Here's how the part is built. I have some questions about the finished solid (model axes, mm). Round coordinates to 2 decimals unless told otherwise and drop trailing zeros. Write each loop counter-clockwise with the first axis right and the second up, starting at its lowest first coordinate (ties: lowest second). Pieces come first, ordered by that corner, then holes. Notation, with made-up numbers: (58.25, 72) - (65.25, 72) arc R19 ccw to (65.25, 85) - close; hole circle Ø1 at (-37, 63.25). An arc over 180 degrees is marked (long way). Use one line per item in the form item = value. Start each with the question number.
1. I want a section at A-A, the plane y = 1.5. List the corners of the cut face in (x, z) for me, plus the area to 3 significant figures.
2. Will this pin go through, and if not, where does the flat tip stop? pin 1 (1.6 mm diameter, centred on x = 1, y = 2, fed in from -Z).
3. If I drill on line 1 along Z through (x, y) = (-2, 2); line 2 along X through (y, z) = (2.7, 2.5); line 3 along Z through (x, y) = (7.5, 0.4), over which ranges is the centre line in solid material (lowest first)?
4. I want a section at B-B, the plane x = 0.5. List the corners of the cut face in (y, z) for me.
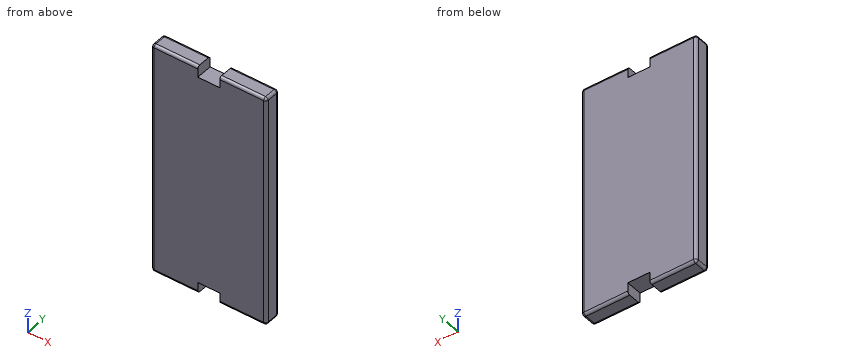
Autodesk Inventor part; units mm, degrees
ref_plane "Плоскость YZ" through (0, 0, 0) normal (1, 0, 0) x (0, 1, 0)
ref_plane "Плоскость XZ" through (0, 0, 0) normal (0, 1, 0) x (-1, 0, 0)
ref_plane "Плоскость XY" through (0, 0, 0) normal (0, 0, 1) x (1, 0, 0)
sketch "Эскиз1" plane through (0, 0, 0) normal (0, 1, 0) x (-1, 0, 0)
  line L0 (10.9667, 22.3) -> (-10.9667, 22.3)
  line L1 (-10.9667, 22.3) -> (-10.9667, -22.3)
  line L2 (-10.9667, -22.3) -> (10.9667, -22.3)
  line L3 (10.9667, -22.3) -> (10.9667, 22.3)
  line L4 (10.9667, 22.3) -> (-10.9667, -22.3) construction
  line L5 (-10.9667, 22.3) -> (10.9667, -22.3) construction
  point P0 (0, 0)
  dimension "d0" = 44.6
  dimension "d1" = 21.9333
extrude "Выдавливание1" add sketch "Эскиз1" along normal blind 3.1
fillet "Сопряжение1" radius 0.5 12 edges at (0, 3.1, 22.3) (0, 0, 22.3) (10.9667, 1.55, 22.3) (-10.9667, 1.55, 22.3) (-10.9667, 3.1, 0) (10.9667, 3.1, 0) (10.9667, 0, 0) (-10.9667, 0, 0) (0, 3.1, -22.3) (0, 0, -22.3) (-10.9667, 1.55, -22.3) (10.9667, 1.55, -22.3)
sketch "Эскиз2" plane through (0, 3.1, 0) normal (0, 1, 0) x (1, 0, 0)
  line L0 (-2.1, 24.4) -> (2.1, 24.4)
  line L1 (2.1, 24.4) -> (2.1, 20.2)
  line L2 (2.1, 20.2) -> (-2.1, 20.2)
  line L3 (-2.1, 20.2) -> (-2.1, 24.4)
  line L4 (10.4667, 22.3) -> (-10.4667, 22.3)
  line L5 (-2.1, 24.4) -> (2.1, 20.2) construction
  line L6 (2.1, 24.4) -> (-2.1, 20.2) construction
  point P0 (0, 0)
  point P1 (0, 22.3)
  dimension "d5" = 4.2
  dimension "d6" = 4.2
extrude "Выдавливание2" cut sketch "Эскиз2" against normal blind 10
mirror "Зеркальное отражение1" about plane through (0, 0, 0) normal (0, 0, 1) of "Выдавливание2"
properties part number "Test2" material "Типовой"
Model answer:
q1.outline = (-10.97, -21.8) arc R0.5 ccw to (-10.47, -22.3) - (-2.1, -22.3) - (-2.1, -20.2) - (2.1, -20.2) - (2.1, -22.3) - (10.47, -22.3) arc R0.5 ccw to (10.97, -21.8) - (10.97, 21.8) arc R0.5 ccw to (10.47, 22.3) - (2.1, 22.3) - (2.1, 20.2) - (-2.1, 20.2) - (-2.1, 22.3) - (-10.47, 22.3) arc R0.5 ccw to (-10.97, 21.8) - close
q1.area = 960 mm2
q2.pin_1 = -20.2
q3.line_1 = -20.2 to 20.2
q3.line_2 = -10.96 to 10.96
q3.line_3 = -22.29 to 22.29
q4.outline = (0, -20.2) - (3.1, -20.2) - (3.1, 20.2) - (0, 20.2) - close
